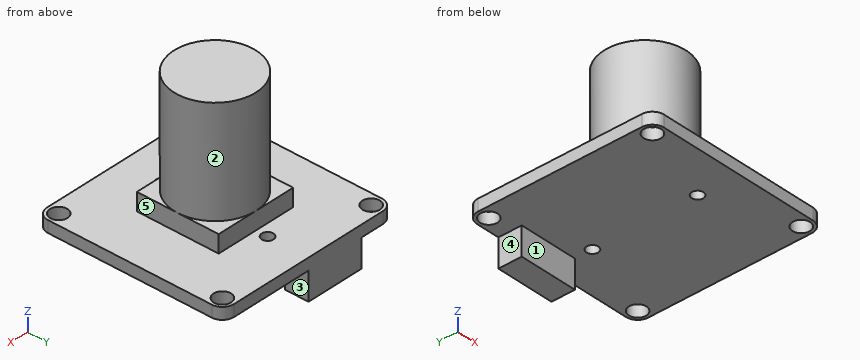
Autodesk Inventor part; units mm, degrees
ref_plane "YZ Plane" through (0, 0, 0) normal (1, 0, 0) x (0, 1, 0)
ref_plane "XZ Plane" through (0, 0, 0) normal (0, 1, 0) x (-1, 0, 0)
ref_plane "XY Plane" through (0, 0, 0) normal (0, 0, 1) x (1, 0, 0)
sketch "스케치1" plane through (0, 0, 0) normal (0, 0, 1) x (1, 0, 0)
  line L0 (-16, 16) -> (16, 16)
  line L1 (16, 16) -> (16, -16)
  line L2 (16, -16) -> (-16, -16)
  line L3 (-16, -16) -> (-16, 16)
  point P0 (0, 0)
  dimension "d0" = 32
  dimension "d1" = 32
  dimension "d2" = 16
  dimension "d3" = 16
extrude "돌출1" add sketch "스케치1" along normal blind 2
sketch "스케치2" plane through (0, 0, 2) normal (0, 0, 1) x (1, 0, 0)
  circle A0 centre (-14, 14) radius 1.5
  circle A1 centre (14, 14) radius 1.5
  circle A2 centre (-14, -14) radius 1.5
  circle A3 centre (14, -14) radius 1.5
  line L0 (-16, 16) -> (-16, -16)
  line L1 (16, 16) -> (-16, 16)
  line L2 (-16, -16) -> (16, -16)
  line L3 (16, -16) -> (16, 16)
  point P0 (0, 0)
  dimension "d6" = 3
  dimension "d7" = 3
  dimension "d8" = 3
  dimension "d9" = 3
  dimension "d10" = 28
  dimension "d12" = 28
  dimension "d13" = 2
  dimension "d14" = 14
  dimension "d15" = 2
  dimension "d16" = 2
  dimension "d17" = 2
  dimension "d18" = 2
  dimension "d19" = 2
  dimension "d20" = 2
extrude "돌출2" cut sketch "스케치2" against normal up to surface (2 mm away) contours A0 | A1 | A2 | A3
sketch "스케치3" plane through (0, 0, 2) normal (0, 0, 1) x (1, 0, 0)
  line L0 (-7, 7) -> (7, 7)
  line L1 (7, 7) -> (7, -7)
  line L2 (7, -7) -> (-7, -7)
  line L3 (-7, -7) -> (-7, 7)
  point P0 (0, 0)
  dimension "d23" = 7
  dimension "d24" = 14
  dimension "d25" = 7
  dimension "d26" = 14
extrude "돌출3" add sketch "스케치3" along normal blind 3
sketch "스케치4" plane through (0, 0, 5) normal (0, 0, 1) x (1, 0, 0)
  circle A0 centre (0, 0) radius 7
  dimension "d29" = 14
extrude "돌출4" add sketch "스케치4" along normal blind 18.2
sketch "스케치6" plane through (0, 0, 2) normal (0, 0, 1) x (1, 0, 0)
  circle A0 centre (0, 9) radius 1
  circle A1 centre (0, -9) radius 1
  line L0 (7, 7) -> (0, 7)
  line L1 (0, -7) -> (7, -7)
  line L2 (-16, 16) -> (-16, -16)
  point P0 (0, 0)
  dimension "d32" = 2
  dimension "d33" = 2
  dimension "d34" = 2
  dimension "d35" = 2
  dimension "d36" = 16
  dimension "d37" = 16
extrude "돌출5" cut sketch "스케치6" against normal up to surface (2 mm away)
sketch "스케치5" plane through (0, 0, 0) normal (0, 0, -1) x (-1, 0, 0)
  line L0 (-16, 16) -> (16, 16)
  line L1 (10, 12) -> (0, 12)
  line L2 (0, 12) -> (0, 16)
  line L3 (0, 16) -> (10, 16)
  line L4 (10, 16) -> (10, 12)
  point P0 (0, 0)
  dimension "d40" = 4
  dimension "d41" = 10
extrude "돌출6" add sketch "스케치5" along normal blind 4.8
fillet "모깎기1" radius 2 4 edges at (-16, -16, 1) (-16, 16, 1) (16, 16, 1) (16, -16, 1)
properties part number "Camera"
Read the model definition and answer for the solid it produces. Units are mm, in the model's axes. Face numbers are marked on the shaded views. A direction names the side the tool comes from. Round coordinates to 2 decimals unless told otherwise and drop trailing zeros. Write each loop counter-clockwise with the first axis right and the second up, starting at its lowest first coordinate (ties: lowest second). Pieces come first, ordered by that corner, then holes. Notation, with made-up numbers: (-16, -9.75) - (18, -9.75) arc R24 ccw to (18, 6.25) - close; hole circle Ø10 at (15, -36). An arc over 180 degrees is marked (long way). One line per question, with ' | ' between items. Start each with the question number.
1. Each of these flat-tipped pins is pushed along its axis until it touches: pin 1 (2.5 mm diameter, centred on x = -2.5, z = 3.5, fed in from +Y); pin 2 (4.5 mm diameter, centred on y = 14, z = -3.5, fed in from -X); pin 3 (2.5 mm diameter, centred on x = 14, y = 14, fed in from +Z); pin 4 (2.5 mm diameter, centred on y = -1.5, z = 3, fed in from -X). Where does it stop, or does it pass through?
2. Find the intervals of material crossed by probe 1 along Y at (x, z) = (14, 1.55); probe 2 along X at (y, z) = (-2.5, 3); probe 3 along Z at (x, y) = (-7, 14), in increasing order. Write a range as [from, to].
3. Section A-A (y = -9) is taken. Determine the outline of the cut face in (x, z).
4. Section C-C (x = -9.5) is taken. Determine the outline of the cut face in (y, z).
5. Section D-D (y = 11.5) is taken. Determine the outline of the cut face in (x, z).
6. Section B-B (x = 13) is taken. Determine the outline of the cut face in (y, z).
7. For the marked faces 1, 2, 3, 4 and 5, determine the directions among +Z, -Z, +X, -X, +Y, -Y from which every point of the face is accessible in a straight line to the end or side of a thin tool.
Filled in:
1) pin 1: y = 7 | pin 2: x = -10 | pin 3: through | pin 4: x = -16
2) probe 1: [-16, -15.5], [-12.5, 12.5], [15.5, 16] | probe 2: [-7, 7] | probe 3: [-4.8, 2]
3) outline: (-16, 0) - (-1, 0) - (-1, 2) - (-16, 2) - close; (1, 0) - (16, 0) - (16, 2) - (1, 2) - close
4) outline: (-16, 0) - (12, 0) - (12, -4.8) - (16, -4.8) - (16, 2) - (-16, 2) - close
5) outline: (-16, 0) - (16, 0) - (16, 2) - (-16, 2) - close
6) outline: (-16, 0) - (-15.12, 0) - (-15.12, 2) - (-16, 2) - close; (-12.88, 0) - (12.88, 0) - (12.88, 2) - (-12.88, 2) - close; (15.12, 0) - (16, 0) - (16, 2) - (15.12, 2) - close
7) face 1: -Z, +X, -X, -Y | face 2: +Z | face 3: -Z, +X, +Y, -Y | face 4: -Z, -X, +Y, -Y | face 5: +Z, +X, +Y, -Y
